Build history of the part. All positions in model axes, mm. A direction names the side the tool comes from. Round coordinates to 2 decimals unless told otherwise and drop trailing zeros. Order: outer loops, then holes, each group sorted by start corner. A loop starts at its lowest first (then second) coordinate and runs counter-clockwise, first axis right, second up. Notation, with made-up numbers: (4, -20.5) -> (11, -20.5) arc R8 ccw to (11, -11.5) -> close; hole circle Ø11 at (-22.5, 16). An arc over 180 degrees is marked (long way). Use a Markdown table: item, result. Add a question column.
Item 1: Slice it at C-C, the plane x = -9. Give the cut face in (y, z), plus the area to 3 significant figures.
Item 2: Pin check, flat tips, straight feed: pin 1 (2 mm diameter, centred on y = -1.5, z = 3.5, fed in from -X); pin 2 (1.9 mm diameter, centred on y = -3.5, z = -26.5, fed in from +X); pin 3 (3 mm diameter, centred on y = -4, z = 35, fed in from -X); pin 4 (8 mm diameter, centred on x = 29, z = -17.5, fed in from +Y). Stop position of each tip, or through.
Item 3: Slice it at B-B, the plane x = 0. Give the cut face in (y, z).
Item 4: 3-axis set-ups, long thin cutter, end or side, ignore diameter. For faces 4 (the face through (-8.04, -3.13, 38.42)), 5 (the face through (29.251, -3, -26)), 6 (the face through (11.673, -3, 34)): which of +Z, -Z, +X, -X, +Y, -Y reach the whole face in a straight line?
Item 5: Two-plate mould, pull along X, no slides. Class faces 1 (the face through (32.87, -3.13, -19.06)), 2 (the face through (-37.37, -3.13, -12.2)), 3 (the face through (8.11, -3.13, 38.46)): released by +X, released by -X, zero draft, split by the parting line, or undercut.
Item 6: Slice it at A-A, the plane z = 0. Give the cut face in (x, y), plus the area to 3 significant figures.
Item 7: Probe L1, parallel to Z at x = 0, y = -4.5; L2, parallel to Z at x = 10, y = -3.5; L3, parallel to X at y = -0.75, z = -16. List the from-to ranges inside material, lowest first.
from build123d import *

# Parameters (mm, degrees)
F0_R     = 11
F1_DEPTH = 6.35
F2_R     = 0.508


with BuildPart() as f1:
    # F0 (on Front) → F1 (new body)
    with BuildSketch(Plane.XZ):
        with BuildLine():
            ThreePointArc((30.936552, -4.382146), (25.241854, -1.227006), (18.736838, -1.490146))
            ThreePointArc((18.736838, -1.490146), (16.277813, 9.398), (8.077915, 16.97165))
            ThreePointArc((8.077915, 16.97165), (11.558309, 22.47359), (11.673226, 28.982913))
            ThreePointArc((11.673226, 28.982913), (9.316126, 33.599741), (5.239277, 36.801355))
            ThreePointArc((5.239277, 36.801355), (0, 37.99832), (-5.239277, 36.801355))
            ThreePointArc((-5.239277, 36.801355), (-9.316126, 33.599741), (-11.673226, 28.982913))
            ThreePointArc((-11.673226, 28.982913), (-11.558309, 22.47359), (-8.077915, 16.97165))
            ThreePointArc((-8.077915, 16.97165), (-16.277813, 9.398), (-18.736838, -1.490146))
            ThreePointArc((-18.736838, -1.490146), (-25.241854, -1.227006), (-30.936552, -4.382146))
            ThreePointArc((-30.936552, -4.382146), (-33.756293, -8.731869), (-34.490547, -13.86333))
            ThreePointArc((-34.490547, -13.86333), (-32.90751, -18.99916), (-29.25127, -22.938025))
            ThreePointArc((-29.25127, -22.938025), (-24.440167, -24.867872), (-19.263326, -24.600767))
            ThreePointArc((-19.263326, -24.600767), (-13.683546, -21.246584), (-10.658923, -15.481504))
            ThreePointArc((-10.658923, -15.481504), (0, -18.796), (10.658923, -15.481504))
            ThreePointArc((10.658923, -15.481504), (13.683546, -21.246584), (19.263326, -24.600767))
            ThreePointArc((19.263326, -24.600767), (24.440167, -24.867872), (29.25127, -22.938025))
            ThreePointArc((29.25127, -22.938025), (32.90751, -18.99916), (34.490547, -13.86333))
            ThreePointArc((34.490547, -13.86333), (33.756293, -8.731869), (30.936552, -4.382146))
        make_face()
        Circle(F0_R, mode=Mode.SUBTRACT)
        with BuildLine():
            Line((40.924496, -10.148688), (30.936552, -4.382146))
            ThreePointArc((30.936552, -4.382146), (33.756293, -8.731869), (34.490547, -13.86333))
            Line((34.490547, -13.86333), (40.924496, -10.148688))
        make_face()
        with BuildLine():
            ThreePointArc((5.239277, 36.801355), (9.316126, 33.599741), (11.673226, 28.982913))
            Line((11.673226, 28.982913), (11.673226, 40.515997))
            Line((11.673226, 40.515997), (5.239277, 36.801355))
        make_face()
        with BuildLine():
            Line((29.25127, -30.367309), (29.25127, -22.938025))
            ThreePointArc((29.25127, -22.938025), (24.440167, -24.867872), (19.263326, -24.600767))
            Line((19.263326, -24.600767), (29.25127, -30.367309))
        make_face()
        with BuildLine():
            ThreePointArc((-11.673226, 28.982913), (-9.316126, 33.599741), (-5.239277, 36.801355))
            Line((-5.239277, 36.801355), (-11.673226, 40.515997))
            Line((-11.673226, 40.515997), (-11.673226, 28.982913))
        make_face()
        with BuildLine():
            Line((-29.25127, -30.367309), (-19.263326, -24.600767))
            ThreePointArc((-19.263326, -24.600767), (-24.440167, -24.867872), (-29.25127, -22.938025))
            Line((-29.25127, -22.938025), (-29.25127, -30.367309))
        make_face()
        with BuildLine():
            ThreePointArc((-34.490547, -13.86333), (-33.756293, -8.731869), (-30.936552, -4.382146))
            Line((-30.936552, -4.382146), (-40.924496, -10.148688))
            Line((-40.924496, -10.148688), (-34.490547, -13.86333))
        make_face()
    extrude(amount=F1_DEPTH)

    # F2
    f2_edges = [f1.edges().sort_by_distance(p)[0] for p in [
        (-11.673226, -3.175, 40.515997),
        (11.673226, -3.175, 40.515997),
        (40.924496, -3.175, -10.148688),
        (29.25127, -3.175, -30.367309),
        (-29.25127, -3.175, -30.367309),
        (-40.924496, -3.175, -10.148688),
    ]]
    fillet(f2_edges, radius=F2_R)


solid = f1.part
Check sheet entries:
| question | item | result |
|---|---|---|
| 1 | outline | (-6.35, -16.5) -> (0, -16.5) -> (0, -6.32) -> (-6.35, -6.32) -> close; (-6.35, 6.32) -> (0, 6.32) -> (0, 16.5) -> (-6.35, 16.5) -> close; (-6.35, 17.9) -> (0, 17.9) -> (0, 38.97) -> (-6.35, 38.97) -> close |
| 1 | area | 263 mm2 |
| 2 | pin 1 | x = -18.63 |
| 2 | pin 2 | x = 29.25 |
| 2 | pin 3 | x = -11.67 |
| 2 | pin 4 | y = 0 |
| 3 | outline | (-6.35, -18.8) -> (0, -18.8) -> (0, -11) -> (-6.35, -11) -> close; (-6.35, 11) -> (0, 11) -> (0, 38) -> (-6.35, 38) -> close |
| 4 | face 4 | +Z, +Y, -Y |
| 4 | face 5 | -Z, +X, +Y, -Y |
| 4 | face 6 | +Z, +X, +Y, -Y |
| 5 | face 1 | released by +X |
| 5 | face 2 | released by -X |
| 5 | face 3 | undercut |
| 6 | outline | (-18.8, -6.35) -> (-11, -6.35) -> (-11, 0) -> (-18.8, 0) -> close; (11, -6.35) -> (18.8, -6.35) -> (18.8, 0) -> (11, 0) -> close |
| 6 | area | 99.0 mm2 |
| 7 | L1 | -18.8 to -11, 11 to 38 |
| 7 | L2 | -15.92 to -4.58, 4.58 to 15.92, 19.18 to 39.55 |
| 7 | L3 | -34.14 to -10.78, -9.86 to 9.86, 10.78 to 34.14 |
